```python
from build123d import *

# Parameters (mm, degrees)
PAD_DEPTH    = 4
SKETCH001_W  = 7
SKETCH001_H  = 7
POCKET_DEPTH = 2


with BuildPart() as part:
    # Sketch → Pad (new body)
    with BuildSketch(Plane.XY):
        with BuildLine():
            ThreePointArc((0, -1.75), (1.75, 0), (0, 1.75))
            Line((0, 11), (0, 1.75))
            Line((7, 11), (0, 11))
            Line((7, -12), (7, 11))
            Line((4.5, -12), (7, -12))
            Line((4.5, -11), (4.5, -12))
            Line((0, -11), (4.5, -11))
            Line((0, -8.75), (0, -11))
            ThreePointArc((0, -8.75), (1.75, -7), (0, -5.25))
            Line((0, -5.25), (0, -1.75))
        make_face()
    pad = extrude(amount=PAD_DEPTH)

    # Sketch001 → Pocket (cut)
    with BuildSketch(Plane.XY):
        with Locations((3.5, 7.5)):
            Rectangle(SKETCH001_W, SKETCH001_H)
    pocket = extrude(amount=POCKET_DEPTH, mode=Mode.SUBTRACT)

    # Mirrored: Pad, Pocket across Sketch V_Axis
    add(pad.mirror(Plane(origin=(0, 0, 0), x_dir=(0, 0, 1), z_dir=(1, 0, 0))))
    add(pocket.mirror(Plane(origin=(0, 0, 0), x_dir=(0, 0, 1), z_dir=(1, 0, 0))), mode=Mode.SUBTRACT)


solid = part.part
```
Input: part model. Units: mm. Frame: model coordinates. Round coordinates to 2 decimals unless told otherwise and drop trailing zeros. Loops run counter-clockwise (first coordinate to the right, second up) from the corner with the lowest first, then second, coordinate; pieces in that order, holes last.
1) Section query C-C on x = -0.25. Return the cut outline in (y, z).
Ans:
outline: (-11, 0) - (-8.73, 0) - (-8.73, 4) - (-11, 4) - close; (-5.27, 0) - (-1.73, 0) - (-1.73, 4) - (-5.27, 4) - close; (1.73, 0) - (4, 0) - (4, 2) - (11, 2) - (11, 4) - (1.73, 4) - close
2) Pull-direction query (X, two-part tool) for faces 1 (the flat face through (6, -12, 2)), 2 (the flat face through (-4.5, -11.5, 2)), 3 (the flat face through (4.5, -11.5, 2)), 4 (the flat face through (7, -3, 2)); classes: released by +X, released by -X, zero draft, split by the parting line, or undercut.
Ans:
face 1: zero draft
face 2: undercut
face 3: undercut
face 4: released by +X
3) Section query B-B on y = 0. Return the cut outline in (x, z), plus the area to 3 significant figures.
Ans:
outline: (-7, 0) - (-1.75, 0) - (-1.75, 4) - (-7, 4) - close; (1.75, 0) - (7, 0) - (7, 4) - (1.75, 4) - close
area: 42.0 mm2
4) Material intervals for line 1 (Y direction, x = -4.25, z = 2.5); line 2 (Z direction, x = 3.25, y = 6.25); line 3 (Y direction, x = -0.5, z = 2.05), sorted ascending.
Ans:
line 1: y = -11 to 11
line 2: z = 2 to 4
line 3: y = -11 to -8.68, -5.32 to -1.68, 1.68 to 11
5) Section query D-D on x = -5. Return the cut outline in (y, z).
Ans:
outline: (-12, 0) - (4, 0) - (4, 2) - (11, 2) - (11, 4) - (-12, 4) - close
6) Section query A-A on z = 1.6. Return the cut outline in (x, y).
Ans:
outline: (-7, -12) - (-4.5, -12) - (-4.5, -11) - (4.5, -11) - (4.5, -12) - (7, -12) - (7, 4) - (-7, 4) - close; hole circle Ø3.5 at (0, -7); hole circle Ø3.5 at (0, 0)
7) Pin query (flat end, axial travel): pin 1 (1.2 mm diameter, centred on x = 3, z = 1.5, fed in from -Y); pin 2 (3.5 mm diameter, centred on x = -2.5, y = 7, fed in from -Z); pin 3 (0.6 mm diameter, centred on x = 4.5, z = 0.5, fed in from +Y). Return the tip coordinate at first contact, or that it passes through.
Ans:
pin 1: stops at y = -11
pin 2: stops at z = 2
pin 3: stops at y = 4
